```python
from build123d import *

# Parameters (mm, degrees)
ESQUISSE3_W             = 200
ESQUISSE3_H             = 200
ESQUISSE3_R             = 5
BOSS_EXTRU_2_DEPTH      = 7
CONG_1_R                = 15
ESQUISSE4_R             = 5
ENL_V_MAT_EXTRU_1_DEPTH = 10


with BuildPart() as part:
    # Esquisse3 → Boss.-Extru.2 (new body)
    with BuildSketch(Plane.XY):
        Rectangle(ESQUISSE3_W, ESQUISSE3_H)
        with Locations((80, 80)):
            Circle(ESQUISSE3_R, mode=Mode.SUBTRACT)
        with Locations((80, -80)):
            Circle(ESQUISSE3_R, mode=Mode.SUBTRACT)
        with Locations((-80, -80)):
            Circle(ESQUISSE3_R, mode=Mode.SUBTRACT)
        with Locations((-80, 80)):
            Circle(ESQUISSE3_R, mode=Mode.SUBTRACT)
    extrude(amount=BOSS_EXTRU_2_DEPTH)

    # Congé1
    cong_1_edges = [part.edges().sort_by_distance(p)[0] for p in [
        (-100, 100, 3.5),
        (100, 100, 3.5),
        (100, -100, 3.5),
        (-100, -100, 3.5),
    ]]
    fillet(cong_1_edges, radius=CONG_1_R)

    # Esquisse4 → Enlèv. mat.-Extru.1 (cut)
    with BuildSketch(Plane(origin=(0, 0, 0), x_dir=(-1, 0, 0), z_dir=(0, 0, -1))):
        with Locations((0, -25)):
            Circle(ESQUISSE4_R)
        with Locations((0, 25)):
            Circle(ESQUISSE4_R)
    extrude(amount=-ENL_V_MAT_EXTRU_1_DEPTH, mode=Mode.SUBTRACT)


solid = part.part
```
Geometry check sheet. Reference: the model listing, model coordinates, mm. Coordinates: 2 decimals unless noted, no trailing zeros. Write each loop counter-clockwise with the first axis right and the second up, starting at its lowest first coordinate (ties: lowest second). Pieces come first, ordered by that corner, then holes. Notation, with made-up numbers: M -36.75,-25 L -24.75,-25 A8 ccw -24.75,-20 Z; hole C 33.5,29.5 d3. An arc over 180 degrees is marked long. One line per item, written item: value. Start each with the question number.
(1) Sectioned sample at D-D, the plane z = 5.25. Enter the section's corners in (x, y).
(2) Sectioned sample at A-A, the plane y = -25. Enter the section's corners in (x, z), and give its area (3 significant figures).
(3) Sectioned sample at B-B, the plane x = 80. Enter the section's corners in (y, z).
(4) Scan lines: line 1 along Y through (x, z) = (-80, 5); line 2 along Y through (x, z) = (0, 3); line 3 along Y through (x, z) = (-86.5, 2.75). Record each from-to range of solid material in increasing order. Write a range as [from, to].
(5) Release check for a two-part mould opening along Y. For faces 1 (the face through (-1, 1, 0)), 2 (the face through (-1, 100, 3)), 3 (the face through (95.49, -95.72, 3.55)), 4 (the face through (84.619, -81.915, 3.451)) record: released by +Y, released by -Y, zero draft, split by the parting line, or undercut.
Filled sheet:
1. outline: M -100,-85 A15 ccw -85,-100 L 85,-100 A15 ccw 100,-85 L 100,85 A15 ccw 85,100 L -85,100 A15 ccw -100,85 Z; hole C -80,-80 d10; hole C -80,80 d10; hole C 0,-25 d10; hole C 0,25 d10; hole C 80,-80 d10; hole C 80,80 d10
2. outline: M -100,0 L -5,0 L -5,7 L -100,7 Z; M 5,0 L 100,0 L 100,7 L 5,7 Z
2. area: 1,330 mm²
3. outline: M -100,0 L -85,0 L -85,7 L -100,7 Z; M -75,0 L 75,0 L 75,7 L -75,7 Z; M 85,0 L 100,0 L 100,7 L 85,7 Z
4. line 1: [-100, -85], [-75, 75], [85, 100]
4. line 2: [-100, -30], [-20, 20], [30, 100]
4. line 3: [-99.92, 99.92]
5. face 1: zero draft
5. face 2: released by +Y
5. face 3: released by -Y
5. face 4: undercut
